```python
from build123d import *

# Parameters (mm, degrees)
SKETCH_1_W          = 40
SKETCH_1_H          = 40
EXTRUDE_1_DEPTH     = 3
SKETCH_2_R          = 2
EXTRUDE_2_DEPTH     = 4.15
SKETCH_4_R          = 2.1
CUT_EXTRUDE_1_DEPTH = 4
SKETCH_3_R          = 1.25
CUT_EXTRUDE_2_DEPTH = 4.15


with BuildPart() as part:
    # 草圖1 → 填料-伸長1 (new body)
    with BuildSketch(Plane.XY):
        Rectangle(SKETCH_1_W, SKETCH_1_H)
    extrude(amount=EXTRUDE_1_DEPTH)

    # 草圖2 → 填料-伸長2 (add)
    with BuildSketch(Plane.XY.offset(3)):
        with Locations((-7.62, 10.795)):
            Circle(SKETCH_2_R)
        with Locations((-7.62, -10.795)):
            Circle(SKETCH_2_R)
        with Locations((7.62, -10.795)):
            Circle(SKETCH_2_R)
        with Locations((7.62, 10.795)):
            Circle(SKETCH_2_R)
    extrude(amount=EXTRUDE_2_DEPTH)

    # 草圖4 → 除料-伸長1 (cut, through all)
    with BuildSketch(Plane.XY.offset(3)):
        with Locations((-15, 15)):
            Circle(SKETCH_4_R)
        with Locations((-15, -15)):
            Circle(SKETCH_4_R)
        with Locations((15, -15)):
            Circle(SKETCH_4_R)
        with Locations((15, 15)):
            Circle(SKETCH_4_R)
    extrude(amount=-CUT_EXTRUDE_1_DEPTH, mode=Mode.SUBTRACT)

    # 草圖3 → 除料-伸長2 (cut)
    with BuildSketch(Plane.XY.offset(7.15)):
        with Locations((-7.62, 10.795)):
            Circle(SKETCH_3_R)
        with Locations((-7.62, -10.795)):
            Circle(SKETCH_3_R)
        with Locations((7.62, -10.795)):
            Circle(SKETCH_3_R)
        with Locations((7.62, 10.795)):
            Circle(SKETCH_3_R)
    extrude(amount=-CUT_EXTRUDE_2_DEPTH, mode=Mode.SUBTRACT)


solid = part.part
```
Geometry: final body of the model. Coordinates: model frame, mm. A direction names the side the tool comes from. Round coordinates to 2 decimals unless told otherwise and drop trailing zeros. Write each loop counter-clockwise with the first axis right and the second up, starting at its lowest first coordinate (ties: lowest second). Pieces come first, ordered by that corner, then holes.
Item 1: Mould query, pull axis Y, two halves, no side actions, for faces 3 (the face through (0, 20, 1)), 4 (the face through (-8.87, -10.74, 5.1)), 5 (the face through (-20, 0, 1)). Classes: +Y half, -Y half, draft (parallel to the pull), parting line (faces both ways), or undercut.
Item 2: Section query A-A (x = -15). Return loops of the section in (y, z).
Item 3: Section query D-D (z = 1.5). Return loops of the section in (x, y).
Item 4: Set-up query: faces 1 (the face through (16.13, 16.77, 1.52)), 2 (the face through (6.37, -10.74, 5.1)). Return all of +Z, -Z, +X, -X, +Y, -Y with unobstructed straight access to the full face (end or side cutting, diameter ignored); none if empty.
Item 5: Pin query (flat end, axial travel): P1, Ø1.2, axis at x = -8, y = -11, coming from the +Z side; P2, Ø3.5, axis at x = 15, y = -15, coming from the -Z side. Return the tip coordinate at first contact, or that it passes through.
Item 6: Material intervals for L1, parallel to Y at x = -7.62, z = 5.3 (3 decimals); L2, parallel to X at y = -14.5, z = 2.5; L3, parallel to Z at x = 5, y = 11, sorted ascending.
Item 7: Section query B-B (z = 5.75). Return loops of the section in (x, y) (3 decimals), plus the area to 3 significant figures.
Completed:
1. face 3: +Y half
1. face 4: undercut
1. face 5: draft
2. outline: (-20, 0) - (-17.1, 0) - (-17.1, 3) - (-20, 3) - close; (-12.9, 0) - (12.9, 0) - (12.9, 3) - (-12.9, 3) - close; (17.1, 0) - (20, 0) - (20, 3) - (17.1, 3) - close
3. outline: (-20, -20) - (20, -20) - (20, 20) - (-20, 20) - close; hole circle Ø4.2 at (-15, -15); hole circle Ø4.2 at (-15, 15); hole circle Ø4.2 at (15, -15); hole circle Ø4.2 at (15, 15)
4. face 1: +Z, -Z
4. face 2: +Z
5. P1: stops at z = 3
5. P2: passes through
6. L1: y = -12.795 to -12.045, -9.545 to -8.795, 8.795 to 9.545, 12.045 to 12.795
6. L2: x = -20 to -17.04, -12.96 to 12.96, 17.04 to 20
6. L3: z = 0 to 3
7. outline: circle Ø4 at (-7.62, -10.795); circle Ø4 at (-7.62, 10.795); circle Ø4 at (7.62, -10.795); circle Ø4 at (7.62, 10.795); hole circle Ø2.5 at (-7.62, -10.795); hole circle Ø2.5 at (-7.62, 10.795); hole circle Ø2.5 at (7.62, -10.795); hole circle Ø2.5 at (7.62, 10.795)
7. area: 30.6 mm2
